from build123d import *

# Parameters (mm, degrees)
F1_DEPTH = 242.57
F2_W     = 6.35
F2_H     = 17.78
F3_DEPTH = 30.683568


with BuildPart() as f1:
    # F0 (on Right) → F1 (new body)
    with BuildSketch(Plane.YZ):
        with BuildLine():
            Line((21.360137, 0), (0, 9.322432))
            Line((0, 9.322432), (0, 30.682568))
            ThreePointArc((0, 30.682568), (-13.802055, 18.43997), (-13.214322, 0))
            Line((-13.214322, 0), (21.360137, 0))
        make_face()
    extrude(amount=F1_DEPTH)

    # F2 (on face) → F3 (cut, through all)
    with BuildSketch(Plane(origin=(0, 0, 0), x_dir=(1, 0, 0), z_dir=(0, 0, -1))):
        with Locations((3.175, -12.470137)):
            Rectangle(F2_W, F2_H)
        with Locations((19.685, -12.470137)):
            Rectangle(F2_W, F2_H)
        with Locations((36.195, -12.470137)):
            Rectangle(F2_W, F2_H)
        with Locations((52.705, -12.470137)):
            Rectangle(F2_W, F2_H)
        with Locations((69.215, -12.470137)):
            Rectangle(F2_W, F2_H)
        with Locations((85.725, -12.470137)):
            Rectangle(F2_W, F2_H)
        with Locations((102.235, -12.470137)):
            Rectangle(F2_W, F2_H)
        with Locations((118.745, -12.470137)):
            Rectangle(F2_W, F2_H)
        with Locations((135.255, -12.470137)):
            Rectangle(F2_W, F2_H)
        with Locations((151.765, -12.470137)):
            Rectangle(F2_W, F2_H)
        with Locations((168.275, -12.470137)):
            Rectangle(F2_W, F2_H)
        with Locations((184.785, -12.470137)):
            Rectangle(F2_W, F2_H)
        with Locations((201.295, -12.470137)):
            Rectangle(F2_W, F2_H)
        with Locations((217.805, -12.470137)):
            Rectangle(F2_W, F2_H)
        with Locations((234.315, -12.470137)):
            Rectangle(F2_W, F2_H)
    extrude(amount=-F3_DEPTH, mode=Mode.SUBTRACT)


solid = f1.part
CAD build for the part. Positions are in the model's coordinates, mm. A direction names the side the tool comes from. Round coordinates to 2 decimals unless told otherwise and drop trailing zeros. Write each loop counter-clockwise with the first axis right and the second up, starting at its lowest first coordinate (ties: lowest second). Pieces come first, ordered by that corner, then holes. Notation, with made-up numbers: M -9.75,82.5 L 25.25,82.5 A30 cw 25.25,117.5 Z; hole C 17,-15.75 d10. An arc over 180 degrees is marked long. Put each result on its own line as item: value. Start each with the question number.
1) Saw through at A-A, the plane y = 6.5. Count the separate pieces of the cut face and the enclosed holes in it, and give its area (3 significant figures).
2) Saw through at B-B, the plane x = 163. Write the cut outline in (y, z), and give its area (3 significant figures).
3) Saw through at C-C, the plane z = 13. Write the cut outline in (x, y).
4) Drill centre lines: probe 1 along Z at (x, y) = (39, -5); probe 2 along Y at (x, z) = (76, 20.5); probe 3 along Y at (x, z) = (159, 29). Where is each one in solid material? Low to high. Write a range as [from, to].
5) Pull direction X, two halves, no side cores. Call faces 1 (the flat face through (120, 0, 0)), 2 (the flat face through (6.35, 9, 2)), 3 (the flat face through (99.06, 9, 2)): pulls with the +X half, pulls with the -X half, needs draft (parallel to the pull), parting line crosses it, or undercut.
6) Pin check, flat tips, straight feed: pin 1 Ø10 at (x, z) = (36.5, 20) entering from -Y; pin 2 Ø2 at (x, z) = (52, 12) entering from +Y; pin 3 Ø8.5 at (y, z) = (13.5, 3.5) entering from -X. Stop position of each tip, or through.
7) 3-axis set-ups, long thin cutter, end or side, ignore diameter. For faces 4 (the flat face through (119.587, 1.336, 8.739)), 5 (the flat face through (82.55, 9, 2)): which of +Z, -Z, +X, -X, +Y, -Y reach the whole face in a straight line?
Resolved:
1. separate pieces: 15
1. enclosed holes: 0
1. area: 955 mm²
2. outline: M -13.21,0 L 21.36,0 L 0,9.32 L 0,30.68 A21.72 ccw Z
2. area: 484 mm²
3. outline: M 0,-15.34 L 242.57,-15.34 L 242.57,0 L 0,0 Z
4. probe 1: [0, 28.49]
4. probe 2: [-12.78, 0]
4. probe 3: [-4.1, 0]
5. face 1: needs draft
5. face 2: pulls with the -X half
5. face 3: undercut
6. pin 1: y = -14.95
6. pin 2: y = 0
6. pin 3: x = 6.35
7. face 4: +Z, +X, -X, +Y
7. face 5: +Z, -Z, +Y
